Verification items for the finished model (mm, model axes). Face numbers are marked on the shaded views. Coordinates: 2 decimals unless noted, no trailing zeros. Write each loop counter-clockwise with the first axis right and the second up, starting at its lowest first coordinate (ties: lowest second). Pieces come first, ordered by that corner, then holes. Notation, with made-up numbers: (57.5, -18) -> (77.5, -18) arc R30 ccw to (77.5, 20) -> close; hole circle Ø1 at (-20, 77.25). An arc over 180 degrees is marked (long way). Answer in a Markdown table with one row per item.
```python
from build123d import *

# Parameters (mm, degrees)
SKETCH_1_W          = 50
SKETCH_1_H          = 40
EXTRUDE_1_DEPTH     = 10
CUT_EXTRUDE_START   = -10
SKETCH_7_W          = 41
SKETCH_7_H          = 26
CUT_EXTRUDE_2_DEPTH = 6
CUT_EXTRUDE_3_DEPTH = 33.57299495


with BuildPart() as part:
    # 草图1 → 凸台-拉伸1 (new body)
    with BuildSketch(Plane(origin=(0, 0, 0), x_dir=(0, 0, -1), z_dir=(0, 1, 0))):
        Rectangle(SKETCH_1_W, SKETCH_1_H)
    extrude(amount=EXTRUDE_1_DEPTH)

    # 草图7 → 切除-拉伸2 (cut)
    with BuildSketch(Plane(origin=(0, 10, 0), x_dir=(0, 0, -1), z_dir=(0, 1, 0)).offset(CUT_EXTRUDE_START)):
        Rectangle(SKETCH_7_W, SKETCH_7_H)
    extrude(amount=CUT_EXTRUDE_2_DEPTH, mode=Mode.SUBTRACT)

    # 草图8 → 切除-拉伸3 (cut, through all)
    with BuildSketch(Plane(origin=(0, 6, 0), x_dir=(0, 0, 1), z_dir=(0, -1, 0))):
        with BuildLine():
            ThreePointArc((-1.5, 0), (-2.290811691, 1.909188309), (-4.2, 2.7))
            Line((-4.2, 2.7), (-4.2, -2.7))
            ThreePointArc((-4.2, -2.7), (-2.290811691, -1.909188309), (-1.5, 0))
        make_face()
        with BuildLine():
            Line((-4.2, -2.7), (-4.2, 2.7))
            ThreePointArc((-4.2, 2.7), (-6.9, 0), (-4.2, -2.7))
        make_face()
        with BuildLine():
            Line((4.2, 2.7), (-4.2, 2.7))
            ThreePointArc((-4.2, 2.7), (-2.290811691, 1.909188309), (-1.5, 0))
            ThreePointArc((-1.5, 0), (-2.290811691, -1.909188309), (-4.2, -2.7))
            Line((-4.2, -2.7), (4.2, -2.7))
            ThreePointArc((4.2, -2.7), (1.5, 0), (4.2, 2.7))
        make_face()
        with BuildLine():
            ThreePointArc((6.9, 0), (6.109188309, 1.909188309), (4.2, 2.7))
            Line((4.2, 2.7), (4.2, -2.7))
            ThreePointArc((4.2, -2.7), (6.109188309, -1.909188309), (6.9, 0))
        make_face()
        with BuildLine():
            Line((4.2, -2.7), (4.2, 2.7))
            ThreePointArc((4.2, 2.7), (1.5, 0), (4.2, -2.7))
        make_face()
    extrude(amount=-CUT_EXTRUDE_3_DEPTH, mode=Mode.SUBTRACT)


solid = part.part
```
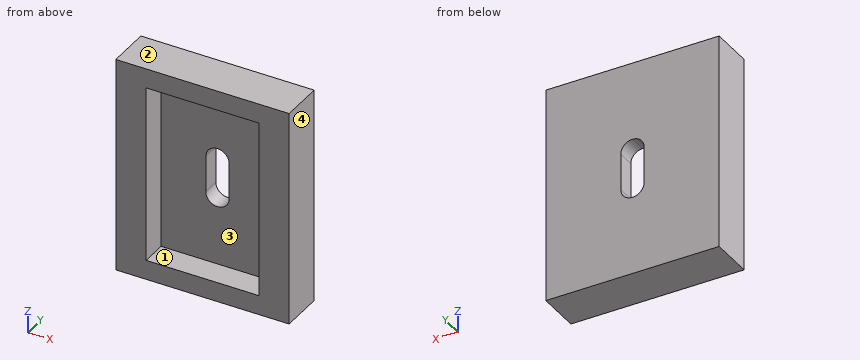
1. Thickness scan on line 1 (X direction, y = 5.75, z = 7); line 2 (X direction, y = 6.75, z = -4); line 3 (Z direction, x = 6, y = 2.5). Record the ranges inside material, lowest first. Write a range as from..to.
Geometry says:
| item | result |
|---|---|
| line 1 | -20..-13, 13..20 |
| line 2 | -20..-2.7, 2.7..20 |
| line 3 | -25..-20.5, 20.5..25 |
2. Depth check by flat-ended pin: P1, Ø8, axis at x = 6.5, z = -8, coming from the -Y side. Enter the tip coordinate at first touch or a pass-through.
Geometry says:
| item | result |
|---|---|
| P1 | y = 6 |
3. Mould release check, pull along X, two halves, no side actions. Record for the marked faces 1, 2, 3 and 4: released by +X, released by -X, zero draft, split by the parting line, or undercut.
Geometry says:
| item | result |
|---|---|
| face 1 | undercut |
| face 2 | zero draft |
| face 3 | undercut |
| face 4 | released by +X |
4. Section check C-C, the plane z = 13.5. Record the boundary of the cut face in (x, y), plus the area to 3 significant figures.
Geometry says:
| item | result |
|---|---|
| outline | (-20, 0) -> (-13, 0) -> (-13, 6) -> (13, 6) -> (13, 0) -> (20, 0) -> (20, 10) -> (-20, 10) -> close |
| area | 244 mm^2 |
5. Section check B-B, the plane x = 12. Record the boundary of the cut face in (y, z).
Geometry says:
| item | result |
|---|---|
| outline | (0, -25) -> (10, -25) -> (10, 25) -> (0, 25) -> (0, 20.5) -> (6, 20.5) -> (6, -20.5) -> (0, -20.5) -> close |
6. Section check A-A, the plane y = 8.5. Record the boundary of the cut face in (x, z).
Geometry says:
| item | result |
|---|---|
| outline | (-20, -25) -> (20, -25) -> (20, 25) -> (-20, 25) -> close; hole (-2.7, -4.2) arc R2.7 ccw to (2.7, -4.2) -> (2.7, 4.2) arc R2.7 ccw to (-2.7, 4.2) -> close |
